Source: CAD feature listing. Evaluate the final solid. Frame: model axes, mm. Face numbers are marked on the shaded views. A direction names the side the tool comes from. Coordinates: 2 decimals unless noted, no trailing zeros. Order: outer loops, then holes, each group sorted by start corner. A loop starts at its lowest first (then second) coordinate and runs counter-clockwise, first axis right, second up.
```python
from build123d import *

# Parameters (mm, degrees)
SKETCH_1_W            = 38
SKETCH_1_H            = 45
EXTRUDE_1_DEPTH       = 3
EXTRUDE_2_DEPTH       = 10
HOLE_WIZARD_3_0_3_1_D = 3
HOLE_WIZARD_3_0_3_2_D = 3
CUT_EXTRUDE_1_DEPTH   = 200
MIRROR_3_COPY_1_DEPTH = 200


with BuildPart() as part:
    # 草图1 → 凸台-拉伸1 (new body)
    with BuildSketch(Plane(origin=(0, 0, 0), x_dir=(1, 0, 0), z_dir=(0, 1, 0))):
        Rectangle(SKETCH_1_W, SKETCH_1_H)
    extrude(amount=EXTRUDE_1_DEPTH)

    # 草图3 → 凸台-拉伸2 (add)
    with BuildSketch(Plane(origin=(0, 0, -5), x_dir=(1, 0, 0), z_dir=(0, 0, -1))):
        Polygon((-5, 0), (-5, 30), (-9, 30), (-9, 10), (-19, 0), align=None)
    extrude_2 = extrude(amount=-EXTRUDE_2_DEPTH)

    # 镜向1: 凸台-拉伸2 across plane
    add(extrude_2.mirror(Plane(origin=(0, 0, 0), x_dir=(0, 0, 1), z_dir=(1, 0, 0))))

    # Ø3.0 (3) 直径孔1 (through all)
    with Locations(Plane(origin=(0, 0, 0), x_dir=(-1, 0, 0), z_dir=(0, -1, 0))):
        with Locations((0, -19), (0, 19)):
            Hole(HOLE_WIZARD_3_0_3_1_D / 2)

    # Ø3.0 (3) 直径孔2 (through all)
    with Locations(Plane(origin=(9, 0, 0), x_dir=(0, 0, -1), z_dir=(1, 0, 0))):
        with Locations((0, -25), (0, -15)):
            Hole(HOLE_WIZARD_3_0_3_2_D / 2)

    # 草图8 → 切除-拉伸1 (cut)
    with BuildSketch(Plane(origin=(0, 0, 0), x_dir=(-1, 0, 0), z_dir=(0, -1, 0))):
        Polygon((19, -5), (5, -22.5), (19, -22.5), align=None)
    cut_extrude_1 = extrude(amount=-CUT_EXTRUDE_1_DEPTH, mode=Mode.SUBTRACT)

    # 镜向2: 切除-拉伸1 across plane
    add(cut_extrude_1.mirror(Plane(origin=(0, 0, 0), x_dir=(0, 0, 1), z_dir=(1, 0, 0))), mode=Mode.SUBTRACT)

    # 镜向3: 切除-拉伸1 across plane
    add(cut_extrude_1.mirror(Plane(origin=(0, 0, 0), x_dir=(1, 0, 0), z_dir=(0, 0, -1))), mode=Mode.SUBTRACT)

    # 镜向3 copy 1 sketch → 镜向3 copy 1 (cut)
    with BuildSketch(Plane.XZ):
        Polygon((19, -5), (5, -22.5), (19, -22.5), align=None)
    extrude(amount=-MIRROR_3_COPY_1_DEPTH, mode=Mode.SUBTRACT)


solid = part.part
```
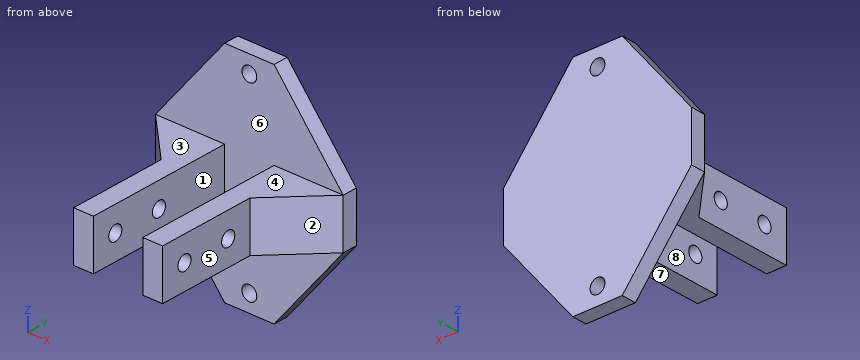
1. Draft query along X for the marked faces 1, 2 and 3. Return one class per face: released by +X, released by -X, zero draft, split by the parting line, or undercut.
Findings:
face 1: undercut
face 2: released by +X
face 3: zero draft
2. Section query D-D on x = 7. Return loops of the section in (y, z).
Findings:
outline: (-30, -5) - (0, -5) - (0, -20) - (3, -20) - (3, 20) - (0, 20) - (0, 5) - (-30, 5) - close; hole circle Ø3 at (-25, 0); hole circle Ø3 at (-15, 0)
3. Access query for the marked faces 4, 5, 6, 7 and 8. Directions: +Z, -Z, +X, -X, +Y, -Y. A direction counts if a zero-diameter tool reaches every point of the face in a straight line with its end or side. Return the directions, or none.
Findings:
face 4: +Z, +X, -X, -Y
face 5: +Z, -Z, +X, -Y
face 6: -Y
face 7: -Z, +X, -X, -Y
face 8: +Z, -Z, -Y
4. Section query A-A on y = -19.5. Return loops of the section in (x, z), plus the area to 3 significant figures.
Findings:
outline: (-9, -5) - (-5, -5) - (-5, 5) - (-9, 5) - close; (5, -5) - (9, -5) - (9, 5) - (5, 5) - close
area: 80.0 mm2
5. Ray query, line 1 (Y direction, x = 6, z = 0); line 2 (Z direction, x = 0, y = 1.25); line 3 (X direction, y = -19.5, z = -1.5). Return the intervals inside material, ascending.
Findings:
line 1: y = -30 to -26.5, -23.5 to -16.5, -13.5 to 3
line 2: z = -22.5 to -20.5, -17.5 to 17.5, 20.5 to 22.5
line 3: x = -9 to -5, 5 to 9
6. Section query C-C on y = -25. Return loops of the section in (x, z), plus the area to 3 significant figures.
Findings:
outline: (-9, -5) - (-5, -5) - (-5, -1.5) - (-9, -1.5) - close; (-9, 1.5) - (-5, 1.5) - (-5, 5) - (-9, 5) - close; (5, -5) - (9, -5) - (9, -1.5) - (5, -1.5) - close; (5, 1.5) - (9, 1.5) - (9, 5) - (5, 5) - close
area: 56.0 mm2
7. Pin query (flat end, axial travel): P1, Ø12, axis at y = -7.5, z = 0.5, coming from the -X side; P2, Ø5, axis at y = -23, z = 2.5, coming from the -X side; P3, Ø6, axis at x = -8.5, y = -17, coming from the -Z side; P4, Ø12, axis at y = -5.5, z = -0.5, coming from the -X side. Return the tip coordinate at first contact, or that it passes through.
Findings:
P1: stops at x = -17.5
P2: stops at x = -9
P3: stops at z = -5
P4: stops at x = -19
8. Section query B-B on z = 0. Return loops of the section in (x, y), plus the area to 3 significant figures.
Findings:
outline: (-19, 0) - (-9, -10) - (-9, -13.5) - (-5, -13.5) - (-5, 0) - (5, 0) - (5, -13.5) - (9, -13.5) - (9, -10) - (19, 0) - (19, 3) - (-19, 3) - close; (-9, -30) - (-5, -30) - (-5, -26.5) - (-9, -26.5) - close; (-9, -23.5) - (-5, -23.5) - (-5, -16.5) - (-9, -16.5) - close; (5, -30) - (9, -30) - (9, -26.5) - (5, -26.5) - close; (5, -23.5) - (9, -23.5) - (9, -16.5) - (5, -16.5) - close
area: 406 mm2
